```python
from build123d import *

# Parameters (mm, degrees)
F0_R     = 41.91
F1_DEPTH = 19.812
F2_R     = 16.637
F3_DEPTH = 1.778
F4_R     = 5.08


with BuildPart() as f1:
    # F0 (on Top) → F1 (new body)
    with BuildSketch(Plane.XY):
        Circle(F0_R)
    extrude(amount=F1_DEPTH)

    # F2 (on face) → F3 (cut)
    with BuildSketch(Plane.XY.offset(19.812)):
        Circle(F2_R)
    extrude(amount=-F3_DEPTH, mode=Mode.SUBTRACT)

    # F4
    f4_edges = [f1.edges().sort_by_distance(p)[0] for p in [
        (-41.91, 0, 0),
        (-41.91, 0, 19.812),
    ]]
    fillet(f4_edges, radius=F4_R)


solid = f1.part
```
For this review, take the finished solid that the model builds, in its own axes (mm). A direction names the side the tool comes from. Round coordinates to 2 decimals unless told otherwise and drop trailing zeros. Loops run counter-clockwise (first coordinate to the right, second up) from the corner with the lowest first, then second, coordinate; pieces in that order, holes last.
(1) Clearance check with flat-ended pins moving along their axes: P1, Ø3, axis at y = 33, z = 10.5, coming from the -X side; P2, Ø1, axis at x = 10.5, z = 3, coming from the +Y side; P3, Ø6, axis at x = -31.5, z = 4, coming from the -Y side; P4, Ø3, axis at x = 4, y = -13, coming from the -Z side. State where each tip first meets the part, or that it passes through.
Returned:
P1: stops at x = -27.64
P2: stops at y = 40.36
P3: stops at y = -30.64
P4: stops at z = 0
(2) Tool access review of faces 1 (the flat face through (-1, 1, 0)), 2 (the flat face through (0, 0, 18.034)): name each direction out of +Z, -Z, +X, -X, +Y, -Y from which nothing blocks a thin tool from reaching the whole face with its end or side.
Returned:
face 1: -Z, +X, -X, +Y, -Y
face 2: +Z
(3) We need section C-C (z = 10). Give the boundary of the cut face in (x, y).
Returned:
outline: circle Ø83.82 at (0, 0)
(4) Mouldability with a two-part tool opening along Y and no side actions: class faces 3 (the cylindrical face through (-2.166, 16.495, 18.935)), 4 (the flat face through (16, -8, 19.812)), 5 (the cylindrical face through (-5.456, 41.553, 9.838)) as released by +Y, released by -Y, zero draft, split by the parting line, or undercut.
Returned:
face 3: undercut
face 4: zero draft
face 5: split by the parting line
(5) Wall thickness on line 1 along Y through (x, z) = (0, 18.5); line 2 along Z through (x, y) = (15.5, 4); line 3 along Y through (x, z) = (0, 18.65): over which ranges is each line inside the solid? List them lowest first.
Returned:
line 1: y = -40.24 to -16.64, 16.64 to 40.24
line 2: z = 0 to 18.03
line 3: y = -40.06 to -16.64, 16.64 to 40.06
(6) We need section D-D (z = 3.25). Give the boundary of the cut face in (x, y).
Returned:
outline: circle Ø83.14 at (0, 0)
(7) We need section A-A (x = 0). Give the boundary of the cut face in (y, z), plus the area to 3 significant figures.
Returned:
outline: (-41.91, 5.08) arc R5.08 ccw to (-36.83, 0) - (36.83, 0) arc R5.08 ccw to (41.91, 5.08) - (41.91, 14.73) arc R5.08 ccw to (36.83, 19.81) - (16.64, 19.81) - (16.64, 18.03) - (-16.64, 18.03) - (-16.64, 19.81) - (-36.83, 19.81) arc R5.08 ccw to (-41.91, 14.73) - close
area: 1,580 mm2
